The listing builds one solid part. Answer for the finished solid, in the listing's coordinates (mm). Round coordinates to 2 decimals unless told otherwise and drop trailing zeros. Order: outer loops, then holes, each group sorted by start corner. A loop starts at its lowest first (then second) coordinate and runs counter-clockwise, first axis right, second up. Notation, with made-up numbers: (15, -12) - (52, -12) arc R23 cw to (52, 2) - close; hole circle Ø11 at (55.5, 59). An arc over 180 degrees is marked (long way). Write item = value, one per line.
from build123d import *

# Parameters (mm, degrees)
SKETCH1_W               = 7.5
SKETCH1_H               = 7.5
SKETCH1_R               = 1.56
BOSS_EXTRUDE1_DEPTH     = 4.9
CUT_EXTRUDE1_DEPTH      = 4.75
CUT_EXTRUDE1_DEPTH_BACK = 4.75


with BuildPart() as part:
    # Sketch1 → Boss-Extrude1 (new body)
    with BuildSketch(Plane.XY):
        Rectangle(SKETCH1_W, SKETCH1_H)
        Circle(SKETCH1_R, mode=Mode.SUBTRACT)
    extrude(amount=BOSS_EXTRUDE1_DEPTH)

    # Sketch5 → Cut-Extrude1 (cut, two sides)
    with BuildSketch(Plane(origin=(0, 0, 0), x_dir=(0, 0, -1), z_dir=(1, 0, 0))) as cut_extrude1_sk:
        Polygon((-2.45, 3.12), (-3.08, 3.75), (-1.82, 3.75), align=None)
    extrude(amount=CUT_EXTRUDE1_DEPTH, mode=Mode.SUBTRACT)
    extrude(cut_extrude1_sk.sketch, amount=-CUT_EXTRUDE1_DEPTH_BACK, mode=Mode.SUBTRACT)


solid = part.part
Q1. Section C-C on z = 3.4 is taken. Determine the outline of the cut face in (x, y), then the cut area to 3 significant figures.
Model answer:
outline = (-3.75, -3.75) - (3.75, -3.75) - (3.75, 3.75) - (-3.75, 3.75) - close; hole circle Ø3.12 at (0, 0)
area = 48.6 mm^2
Q2. A flat-ended cylindrical pin translates along its axis: P1, Ø2, axis at x = -1.5, y = -1.5, coming from the -Z side. Find the tip coordinate at first contact, or state that the pin passes through.
Model answer:
P1 = 0
Q3. Section A-A on y = 0 is taken. Determine the outline of the cut face in (x, z), then the cut area to 3 significant figures.
Model answer:
outline = (-3.75, 0) - (-1.56, 0) - (-1.56, 4.9) - (-3.75, 4.9) - close; (1.56, 0) - (3.75, 0) - (3.75, 4.9) - (1.56, 4.9) - close
area = 21.5 mm^2
Q4. Section B-B on x = 0 is taken. Determine the outline of the cut face in (y, z), then the cut area to 3 significant figures.
Model answer:
outline = (-3.75, 0) - (-1.56, 0) - (-1.56, 4.9) - (-3.75, 4.9) - close; (1.56, 0) - (3.75, 0) - (3.75, 1.82) - (3.12, 2.45) - (3.75, 3.08) - (3.75, 4.9) - (1.56, 4.9) - close
area = 21.1 mm^2
Q5. Find the intervals of material crossed by line 1 (Y direction, x = 0, z = 3.1); line 2 (X direction, y = 0.25, z = 4.1); line 3 (Y direction, x = -1, z = 3.9), in increasing order. Write a range as from..to.
Model answer:
line_1 = -3.75..-1.56, 1.56..3.75
line_2 = -3.75..-1.54, 1.54..3.75
line_3 = -3.75..-1.2, 1.2..3.75
Q6. Section D-D on y = -1 is taken. Determine the outline of the cut face in (x, z), then the cut area to 3 significant figures.
Model answer:
outline = (-3.75, 0) - (-1.2, 0) - (-1.2, 4.9) - (-3.75, 4.9) - close; (1.2, 0) - (3.75, 0) - (3.75, 4.9) - (1.2, 4.9) - close
area = 25.0 mm^2
